Autodesk Inventor part; units mm, degrees
ref_plane "YZ Plane" through (0, 0, 0) normal (1, 0, 0) x (0, 1, 0)
ref_plane "XZ Plane" through (0, 0, 0) normal (0, 1, 0) x (-1, 0, 0)
ref_plane "XY Plane" through (0, 0, 0) normal (0, 0, 1) x (1, 0, 0)
sketch "Skizze1" plane through (0, 0, 0) normal (0, 0, 1) x (1, 0, 0)
  line L0 (7.75, -17.6806) -> (7.75, 17.6806)
  line L1 (-7.75, 17.6806) -> (-7.75, -17.6806)
  circle A0 centre (0, 0) radius 3.025
  arc A1 (-5.3363, -21.3526) -> (5.3363, -21.3526) centre (0, -9) ccw
  arc A2 (5.3363, -21.3526) -> (7.75, -17.6806) centre (3.75, -17.6806) ccw
  arc A3 (7.75, 17.6806) -> (5.3363, 21.3526) centre (3.75, 17.6806) ccw
  arc A4 (5.3363, 21.3526) -> (-5.3363, 21.3526) centre (0, 9) ccw
  arc A5 (-5.3363, 21.3526) -> (-7.75, 17.6806) centre (-3.75, 17.6806) ccw
  arc A6 (-7.75, -17.6806) -> (-5.3363, -21.3526) centre (-3.75, -17.6806) ccw
  circle A7 centre (-0.25, 17) radius 1.7
  circle A8 centre (-0.25, -7) radius 1.7
  line L2 (5.34, 14.1) -> (3.3, 14.1)
  line L3 (3.3, 14.1) -> (3.3, 17.74)
  line L4 (3.3, 17.74) -> (5.34, 17.74)
  line L5 (5.34, 17.74) -> (5.34, 14.1)
  line L6 (-3.8, 14.1) -> (-5.84, 14.1)
  line L7 (-5.84, 14.1) -> (-5.84, 17.74)
  line L8 (-5.84, 17.74) -> (-3.8, 17.74)
  line L9 (-3.8, 17.74) -> (-3.8, 14.1)
  circle A9 centre (-0.25, -15.278) radius 2.9
  point P0 (0, 0)
  point P1 (-17.1225, -5.975)
  point P2 (-17.1225, -12.025)
  point P3 (-17.1225, 6.3)
  point P4 (-17.1225, -14.3)
  point P5 (-17.1225, -17.7)
extrude "Extrusion1" add sketch "Skizze1" along normal blind 4 contours A2 A1 A6 L1 A5 A4 A3 L0 | A0 | A7 | A8 | L2 L3 L4 L5 | L6 L7 L8 L9 | A9
sketch "Skizze2" plane through (0, 0, 0) normal (0, 0, -1) x (-1, 0, 0)
  circle A0 centre (0, 0) radius 3.025
  arc A1 (-5.3363, -21.3526) -> (5.3363, -21.3526) centre (0, -9) ccw
  arc A2 (-7.75, -17.6806) -> (-5.3363, -21.3526) centre (-3.75, -17.6806) ccw
  line L0 (-7.75, -17.6806) -> (-7.75, 17.6806)
  arc A3 (-5.3363, 21.3526) -> (-7.75, 17.6806) centre (-3.75, 17.6806) ccw
  arc A4 (5.3363, 21.3526) -> (-5.3363, 21.3526) centre (0, 9) ccw
  arc A5 (7.75, 17.6806) -> (5.3363, 21.3526) centre (3.75, 17.6806) ccw
  line L1 (7.75, 17.6806) -> (7.75, -17.6806)
  arc A6 (5.3363, -21.3526) -> (7.75, -17.6806) centre (3.75, -17.6806) ccw
  circle A7 centre (0.25, 17) radius 1.7
  circle A8 centre (0.25, -7) radius 1.7
  line L2 (-5.34, 14.1) -> (-3.3, 14.1)
  line L3 (-3.3, 14.1) -> (-3.3, 17.74)
  line L4 (-3.3, 17.74) -> (-5.34, 17.74)
  line L5 (-5.34, 17.74) -> (-5.34, 14.1)
  line L6 (3.8, 14.1) -> (5.84, 14.1)
  line L7 (5.84, 14.1) -> (5.84, 17.74)
  line L8 (5.84, 17.74) -> (3.8, 17.74)
  line L9 (3.8, 17.74) -> (3.8, 14.1)
  circle A9 centre (0.25, -15.278) radius 2.9
  point P0 (0, 0)
extrude "Extrusion2" cut sketch "Skizze2" against normal blind 3.1 contours A0
sketch "Skizze3" plane through (0, 0, 0) normal (0, 0, -1) x (-1, 0, 0)
  circle A0 centre (0, 0) radius 3.025
  arc A1 (-5.3363, -21.3526) -> (5.3363, -21.3526) centre (0, -9) ccw
  arc A2 (-7.75, -17.6806) -> (-5.3363, -21.3526) centre (-3.75, -17.6806) ccw
  line L0 (-7.75, -17.6806) -> (-7.75, 17.6806)
  arc A3 (-5.3363, 21.3526) -> (-7.75, 17.6806) centre (-3.75, 17.6806) ccw
  arc A4 (5.3363, 21.3526) -> (-5.3363, 21.3526) centre (0, 9) ccw
  arc A5 (7.75, 17.6806) -> (5.3363, 21.3526) centre (3.75, 17.6806) ccw
  line L1 (7.75, 17.6806) -> (7.75, -17.6806)
  arc A6 (5.3363, -21.3526) -> (7.75, -17.6806) centre (3.75, -17.6806) ccw
  circle A7 centre (0.25, 17) radius 1.7
  circle A8 centre (0.25, -7) radius 1.7
  line L2 (-5.34, 14.1) -> (-3.3, 14.1)
  line L3 (-3.3, 14.1) -> (-3.3, 17.74)
  line L4 (-3.3, 17.74) -> (-5.34, 17.74)
  line L5 (-5.34, 17.74) -> (-5.34, 14.1)
  line L6 (3.8, 14.1) -> (5.84, 14.1)
  line L7 (5.84, 14.1) -> (5.84, 17.74)
  line L8 (5.84, 17.74) -> (3.8, 17.74)
  line L9 (3.8, 17.74) -> (3.8, 14.1)
  circle A9 centre (0.25, -15.278) radius 2.9
  point P0 (0, 0)
hole "Bohrung1" at (-0.25, 17, 0) at (-0.25, -7, 0) direction (0, 0, 1) diameter 5.6 depth 3.2 counterbore diameter 7.1 counterbore depth 1.2
sketch "Skizze4" plane through (0, 0, 4) normal (0, 0, 1) x (1, 0, 0)
  circle A0 centre (-0.25, 17) radius 3.55
  circle A1 centre (-0.25, -7) radius 3.55
  circle A2 centre (0, 0) radius 3.025
  arc A3 (5.3363, -21.3526) -> (7.75, -17.6806) centre (3.75, -17.6806) ccw
  arc A4 (-5.3363, -21.3526) -> (5.3363, -21.3526) centre (0, -9) ccw
  arc A5 (-7.75, -17.6806) -> (-5.3363, -21.3526) centre (-3.75, -17.6806) ccw
  line L0 (-7.75, 17.6806) -> (-7.75, -17.6806)
  arc A6 (-5.3363, 21.3526) -> (-7.75, 17.6806) centre (-3.75, 17.6806) ccw
  arc A7 (5.3363, 21.3526) -> (-5.3363, 21.3526) centre (0, 9) ccw
  arc A8 (7.75, 17.6806) -> (5.3363, 21.3526) centre (3.75, 17.6806) ccw
  line L1 (7.75, -17.6806) -> (7.75, 17.6806)
  circle A9 centre (12.6079, -10) radius 2.8
  circle A10 centre (12.6079, -10) radius 2.8
  line L2 (4.1087, 0) -> (7.1087, 0)
  line L3 (7.1087, 0) -> (2.8877, -6.1994)
  line L4 (2.8877, -6.1994) -> (-0.1123, -6.1994)
  line L5 (-0.1123, -6.1994) -> (4.1087, 0)
  line L6 (2.721, 6.1994) -> (5.721, 6.1994)
  line L7 (5.721, 6.1994) -> (-2.721, -6.1994)
  line L8 (-2.721, -6.1994) -> (-5.721, -6.1994)
  line L9 (-5.721, -6.1994) -> (2.721, 6.1994)
  line L10 (-2.8877, 6.1994) -> (0.1123, 6.1994)
  line L11 (0.1123, 6.1994) -> (-4.1087, 0)
  line L12 (-4.1087, 0) -> (-7.1087, 0)
  line L13 (-7.1087, 0) -> (-2.8877, 6.1994)
  line L14 (7.1087, 6.1994) -> (7.1087, -6.1994)
  line L15 (7.1087, -6.1994) -> (-7.1087, -6.1994)
  line L16 (-7.1087, -6.1994) -> (-7.1087, 6.1994)
  line L17 (-7.1087, 6.1994) -> (7.1087, 6.1994)
  point P0 (0, 0)
  point P1 (16.5579, -10)
  point P2 (16.5579, -10)
  point P3 (16.5579, -10)
  point P4 (50.5428, -9.282)
  point P5 (-4.221, -6.1994)
  point P6 (4.221, 6.1994)
  point P7 (-1.3877, 6.1994)
  point P8 (1.3877, -6.1994)
  dimension "d89" = 5.6
  dimension "d104" = 5.6
  dimension "d107" = 14.2174
  dimension "d108" = 12.3988
  dimension "d109" = 2.1563
  dimension "d110" = 2.1563
  dimension "d111" = 2.4798
  dimension "d112" = 2.4798
  dimension "d113" = 2.4798
  dimension "d114" = 6.1994
  dimension "d115" = 6.1994
  dimension "d116" = 6.1994
  dimension "d117" = 15.5
  dimension "d118" = 0.6413
move faces "Verschieben1" translate (0, 0, 0.5) faces at (-2.5833, -5.8935, 4)
extrude "Extrusion4" cut sketch "Skizze4" along normal mid plane 0.8 contours L8 L9 A2 L7 A1 | A1 L7 L8 | L3 L4 L5 A1 | A1 L5 L2 L3 | A2 L9 L7 | A2 L9 L6 L7 | L13 L10 L11 L12
extrude "Extrusion5" cut sketch "Skizze4" along normal through all contours L8 L9 A2 L7 A1 | A1 L7 L8 | L3 L4 L5 A1 | A1 L5 L2 L3 | A2 L9 L7 | A2 L9 L6 L7 | L13 L10 L11 L12
sketch "Skizze5" plane through (0, 0, 0) normal (0, 0, -1) x (-1, 0, 0)
  circle A0 centre (0.25, -15.278) radius 2.9
  point P0 (0, 0)
extrude "Extrusion6" cut sketch "Skizze5" against normal blind 1.4
chamfer "Fase2" distance 0.2 distance2 0.8 1 edges at (-0.25, -10.55, 0) measured on face at (6.175, 0, 0)
chamfer "Fase3" distance 2 distance2 0.4 1 edges at (-0.25, -9.8, 1.2) measured on face at (0.1992, -4.2363, 2.5333)
chamfer "Fase4" distance 2 distance2 0.4 1 edges at (-0.25, 14.2, 1.2) measured on face at (0.1992, 19.7637, 2.5333)
chamfer "Fase5" distance 0.2 distance2 0.8 1 edges at (-0.25, 13.45, 0) measured on face at (6.175, 0, 0)
chamfer "Fase6" distance 0.4 angle 45 8 edges at (-7.75, 0, 0) (-7.0925, -19.8777, 0) (0, -22.4559, 0) (7.0925, -19.8777, 0) (7.75, 0, 0) (7.0925, 19.8777, 0) (0, 22.4559, 0) (-7.0925, 19.8777, 0)
chamfer "Fase7" distance 2 angle 45 8 edges at (7.75, 0, 4.5) (7.0925, 19.8777, 4.5) (0, 22.4559, 4.5) (-7.0925, 19.8777, 4.5) (-7.75, 0, 4.5) (-7.0925, -19.8777, 4.5) (0, -22.4559, 4.5) (7.0925, -19.8777, 4.5)
properties part number "Cover_Angled"
The model under review builds one solid part; all positions refer to its coordinate system, in mm. A direction names the side the tool comes from. Coordinates: 2 decimals unless noted, no trailing zeros. Loops run counter-clockwise (first coordinate to the right, second up) from the corner with the lowest first, then second, coordinate; pieces in that order, holes last. Notation, with made-up numbers: M 33.5,27 L 40.5,27 A25 ccw 40.5,57 Z; hole C 77,-18.5 d10. An arc over 180 degrees is marked long. Put each result on its own line as item: value. Start each with the question number.
Q1. The part is to be moulded in two halves that separate along Y. For faces 1 (the flat face through (-7.75, 0, 1)), 2 (the flat face through (4, 6.199, 4)), 3 (the cylindrical face through (-0.077, 22.456, 1.435)), say which applies: +Y half, -Y half, draft (parallel to the pull), parting line (faces both ways), or undercut.
Q2. For faces 4 (the cylindrical face through (7.075, 19.905, 1.435)), 5 (the flat face through (0, 0, 3.6)), 6 (the flat face through (0, 17, 3.2)), 7 (the cylindrical face through (0.077, -22.456, 1.435)), 8 (the flat face through (5, 0, 4)), list the 3-axis set-ups (+Z, -Z, +X, -X, +Y, -Y) from which the entire face can be reached by the end or side of a thin tool; tool diameter is ignored.
Q3. Add section B-B (z = 1.8). Write out the cut boundary in (x, y) (3 decimals).
Q4. Wall thickness on line 1 (Y direction, x = -0.25, z = 1.1); line 2 (Y direction, x = 0.75, z = 2.9); line 3 (X direction, y = 17, z = 0.95): over which ranges is each line inside the solid? List them lowest first.
Q5. Clearance check with flat-ended pins moving along their axes: pin 1 (1.8 mm diameter, centred on x = -1, y = 1, fed in from -Z); pin 2 (1 mm diameter, centred on x = 3.5, z = 4, fed in from -Y); pin 3 (0.7 mm diameter, centred on x = 6, z = 4, fed in from -Y). State where each tip first meets the part, or that it passes through.
Answers:
1. face 1: draft
1. face 2: undercut
1. face 3: +Y half
2. face 4: +Z, -Z, +X, +Y
2. face 5: +Z
2. face 6: -Z
2. face 7: +Z, -Z, -Y
2. face 8: +Z, +X
3. outline: M -7.75,-17.681 A4 ccw -5.336,-21.353 A13.456 ccw 5.336,-21.353 A4 ccw 7.75,-17.681 L 7.75,17.681 A4 ccw 5.336,21.353 A13.456 ccw -5.336,21.353 A4 ccw -7.75,17.681 Z; hole C -0.25,-7 d6.16; hole C -0.25,17 d6.16; hole C 0,0 d6.05
4. line 1: y = -22.45 to -18.18, -12.38 to -10.55, -3.45 to -3.01, 3.01 to 13.45, 20.55 to 22.45
4. line 2: y = -22.03 to -9.68, -4.32 to -2.93, 2.93 to 14.32, 19.68 to 22.03
4. line 3: x = -7.75 to -3.8, 3.3 to 7.75
5. pin 1: stops at z = 3.1
5. pin 2: stops at y = -20.97
5. pin 3: stops at y = -19.57
